from build123d import *

# Parameters (mm, degrees)
SKETCH1_R           = 14.2875
SKETCH1_R_2         = 2.54
BOSS_EXTRUDE1_DEPTH = 3.175
CUT_EXTRUDE1_DEPTH  = 162.674043733
FILLET3_R           = 6.35
SKETCH3_R           = 2.54
BOSS_EXTRUDE3_DEPTH = 3.175
SKETCH6_R           = 2.54
BOSS_EXTRUDE4_DEPTH = 3.175
FILLET2_R           = 6.35
CUT_EXTRUDE2_DEPTH  = 169.237022961
CUT_EXTRUDE3_DEPTH  = 169.237022961
CUT_EXTRUDE4_DEPTH  = 168.265702461
SKETCH15_R          = 2.54
BOSS_EXTRUDE8_DEPTH = 3.175
FILLET4_R           = 2.54


with BuildPart() as part:
    # Sketch1 → Boss-Extrude1 (new body)
    with BuildSketch(Plane.XY):
        with BuildLine():
            Line((-8.89, 25.4), (8.89, 25.4))
            ThreePointArc((8.89, 25.4), (17.870256121, 21.680256121), (21.59, 12.7))
            Line((21.59, 12.7), (21.59, -117.775079775))
            ThreePointArc((21.59, -117.775079775), (21.127743647, -120.388718212), (19.797058824, -122.685251408))
            Line((19.797058824, -122.685251408), (-7.952696208, -155.616779465))
            ThreePointArc((-7.952696208, -155.616779465), (-12.268297602, -157.851943494), (-16.900388255, -156.380852124))
            Line((-16.900388255, -156.380852124), (-32.439211784, -143.287061102))
            ThreePointArc((-32.439211784, -143.287061102), (-34.674375812, -138.971459708), (-33.203284443, -134.339369055))
            Line((-33.203284443, -134.339369055), (-23.382941176, -122.685251408))
            ThreePointArc((-23.382941176, -122.685251408), (-22.052256353, -120.388718212), (-21.59, -117.775079775))
            Line((-21.59, -117.775079775), (-21.59, 12.7))
            ThreePointArc((-21.59, 12.7), (-17.870256121, 21.680256121), (-8.89, 25.4))
        make_face()
        Circle(SKETCH1_R, mode=Mode.SUBTRACT)
        with Locations((0, -101.6)):
            Circle(SKETCH1_R, mode=Mode.SUBTRACT)
        with Locations((-18.532085478, -142.550133084)):
            Circle(SKETCH1_R_2, mode=Mode.SUBTRACT)
        with Locations((0, -50.8)):
            Circle(SKETCH1_R_2, mode=Mode.SUBTRACT)
    extrude(amount=BOSS_EXTRUDE1_DEPTH)

    # Sketch2 → Cut-Extrude1 (cut, through all)
    with BuildSketch(Plane.XY):
        with BuildLine():
            ThreePointArc((19.159083004, -91.647229609), (9.182340769, -50.8), (19.159083004, -9.952770391))
            ThreePointArc((19.159083004, -9.952770391), (20.973467787, -5.122670102), (21.59, 0))
            Line((21.59, 0), (27.94, 0))
            Line((27.94, 0), (27.94, -121.656687185))
            Line((27.94, -121.656687185), (-7.620284479, -163.8572221))
            Line((-7.620284479, -163.8572221), (-17.501317584, -155.874478972))
            Line((-17.501317584, -155.874478972), (16.51, -115.512152961))
            ThreePointArc((16.51, -115.512152961), (20.280273667, -109.005308906), (21.59, -101.6))
            ThreePointArc((21.59, -101.6), (20.973467787, -96.477329898), (19.159083004, -91.647229609))
        make_face()
        with BuildLine():
            Line((-21.59, -41.275), (-21.59, -60.325))
            ThreePointArc((-21.59, -60.325), (-12.065, -50.8), (-21.59, -41.275))
        make_face()
    extrude(amount=CUT_EXTRUDE1_DEPTH, mode=Mode.SUBTRACT)


with BuildPart() as cut_extrude1_piece_1:
    # of the separate pieces the step leaves, piece 1, a body of its own (cut_extrude1_pieces)
    add(part.part.solids().sort_by_distance((-8.89, 25.4, 0))[0])

    # Fillet3
    fillet3_edges = [cut_extrude1_piece_1.edges().sort_by_distance(p)[0] for p in [
        (-21.59, -41.275, 1.5875),
        (-21.59, -60.325, 1.5875),
    ]]
    fillet(fillet3_edges, radius=FILLET3_R)

    # Sketch3 → Boss-Extrude3 (add)
    with BuildSketch(Plane.XY.offset(3.175)):
        with BuildLine():
            Line((-27.351416194, -127.394768527), (-36.025496499, -137.688579))
            ThreePointArc((-36.025496499, -137.688579), (-37.217489152, -141.441859142), (-35.4063854, -144.93869507))
            Line((-35.4063854, -144.93869507), (-24.403104784, -154.210610454))
            ThreePointArc((-24.403104784, -154.210610454), (-19.771014132, -155.681701823), (-15.455412737, -153.446537795))
            Line((-15.455412737, -153.446537795), (-7.557639641, -144.073996091))
            Line((-7.557639641, -144.073996091), (-27.351416194, -127.394768527))
        make_face()
        with Locations((-18.532085478, -142.550133084)):
            Circle(SKETCH3_R, mode=Mode.SUBTRACT)
    extrude(amount=-BOSS_EXTRUDE3_DEPTH)

    # Sketch6 → Boss-Extrude4 (add)
    with BuildSketch(Plane.XY.offset(3.175)):
        Polygon((-35.4063854, -144.93869507), (-63.620410749, -121.164144113), (-51.344981666, -106.596497054), (-27.065569901, -127.055545526), align=None)
        with Locations((-52.626813855, -117.972130278)):
            Circle(SKETCH6_R, mode=Mode.SUBTRACT)
    extrude(amount=-BOSS_EXTRUDE4_DEPTH)

    # Fillet2
    fillet2_edges = [cut_extrude1_piece_1.edges().sort_by_distance(p)[0] for p in [
        (-63.620410749, -121.164144113, 1.5875),
        (-51.344981666, -106.596497054, 1.5875),
        (-27.065569901, -127.055545526, 1.5875),
    ]]
    fillet(fillet2_edges, radius=FILLET2_R)

    # Sketch7 → Cut-Extrude2 (cut, through all)
    with BuildSketch(Plane.XY.offset(3.175)):
        with BuildLine():
            Line((-21.59, 0), (-21.59, 31.75))
            Line((-21.59, 31.75), (21.59, 31.75))
            Line((21.59, 31.75), (21.59, 0))
            ThreePointArc((21.59, 0), (0, 21.59), (-21.59, 0))
        make_face()
    extrude(amount=-CUT_EXTRUDE2_DEPTH, mode=Mode.SUBTRACT)


with BuildPart() as cut_extrude1_piece_2:
    # of the separate pieces the step leaves, piece 2, a body of its own (cut_extrude1_pieces)
    add(part.part.solids().sort_by_distance((-16.900388255, -156.380852124, 0))[0])


with BuildPart() as cut_extrude3_tool:
    # Sketch10 → Cut-Extrude3 (new, through all)
    with BuildSketch(Plane.XY.offset(3.175)):
        with BuildLine():
            Line((-18.151882461, -155.32628042), (-17.361482582, -157.512020269))
            Line((-17.361482582, -157.512020269), (-14.375706423, -156.432313955))
            Line((-14.375706423, -156.432313955), (-15.455412737, -153.446537795))
            ThreePointArc((-15.455412737, -153.446537795), (-16.679911193, -154.563907595), (-18.151882461, -155.32628042))
        make_face()
    extrude(amount=-CUT_EXTRUDE3_DEPTH)


with BuildPart() as cut_extrude1_piece_1_1:
    add(cut_extrude1_piece_1.part)

    # Cut-Extrude3: cut by cut_extrude3_tool
    add(cut_extrude3_tool.part, mode=Mode.SUBTRACT)

    # Sketch12 → Cut-Extrude4 (cut, through all)
    with BuildSketch(Plane.XY.offset(3.175)):
        with BuildLine():
            Line((-21.59, -101.6), (-72.39, -101.6))
            Line((-72.39, -101.6), (-72.39, -165.1))
            Line((-72.39, -165.1), (16.51, -165.1))
            Line((16.51, -165.1), (16.51, -115.512152961))
            ThreePointArc((16.51, -115.512152961), (-7.405308906, -121.880273667), (-21.59, -101.6))
        make_face()
    extrude(amount=-CUT_EXTRUDE4_DEPTH, mode=Mode.SUBTRACT)

    # Sketch15 → Boss-Extrude8 (add)
    with BuildSketch(Plane.XY.offset(3.175)):
        with BuildLine():
            ThreePointArc((-34.29, -3.81), (-30.887045256, -16.51), (-21.59, -25.807045256))
            Line((-21.59, -25.807045256), (-21.59, 0))
            ThreePointArc((-21.59, 0), (-15.266435406, 15.266435406), (0, 21.59))
            Line((0, 21.59), (-8.89, 21.59))
            ThreePointArc((-8.89, 21.59), (-26.850512242, 14.150512242), (-34.29, -3.81))
        make_face()
        with Locations((-24.765, -3.81)):
            Circle(SKETCH15_R, mode=Mode.SUBTRACT)
    extrude(amount=-BOSS_EXTRUDE8_DEPTH)

    # Fillet4
    fillet4_edges = [cut_extrude1_piece_1_1.edges().sort_by_distance(p)[0] for p in [
        (-21.59, -25.807045256, 1.5875),
    ]]
    fillet(fillet4_edges, radius=FILLET4_R)


with BuildPart() as cut_extrude1_piece_2_1:
    add(cut_extrude1_piece_2.part)

    # Cut-Extrude3: cut by cut_extrude3_tool
    add(cut_extrude3_tool.part, mode=Mode.SUBTRACT)


solid = cut_extrude1_piece_1_1.part
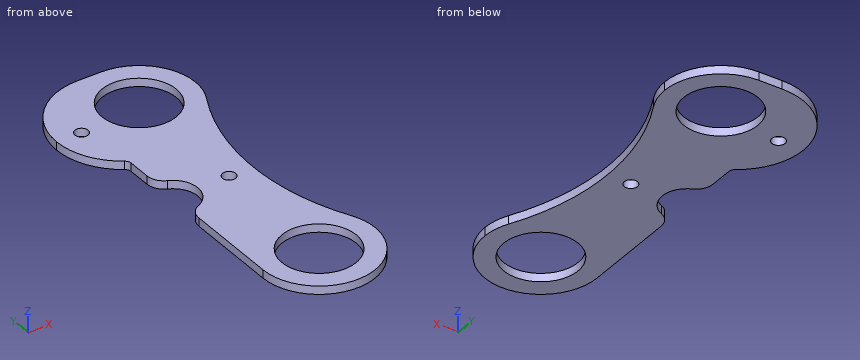
Geometry: final body of the model. Coordinates: model frame, mm. Give positions to 0.01 mm unless a question says otherwise; leave off trailing zeros. Write each loop counter-clockwise with the first axis right and the second up, starting at its lowest first coordinate (ties: lowest second). Pieces come first, ordered by that corner, then holes. Notation, with made-up numbers: M 78,86.25 L 91,86.25 A17 ccw 91,98.25 Z; hole C 1.25,-23.5 d11. An arc over 180 degrees is marked long. Answer in a Markdown table with one row per item. Add a question column.
(1) Section C-C on x = -7.5. Return loops of the section in (y, z) (3 decimals), and give its area (3 significant figures).
(2) Section B-B on z = 2.45. State how many separate pieces and enclosed holes the cut face has, and give its area (3 significant figures).
(3) Ray query, line 1 (Y direction, x = -5.5, z = 0.25); line 2 (Y direction, x = 8, z = 2.4); line 3 (Y direction, x = -19, z = 1.3). Return the intervals inside material, ascending.
(4) Section D-D on x = 5. Return loops of the section in (y, z) (3 decimals).
(5) Section A-A on y = -50.8. Return loops of the section in (x, z) (3 decimals), and give its area (3 significant figures).
(6) First-contact query: pin 1 (1 mm diameter, centred on y = -34.5, z = 1.5, fed in from +X); pin 2 (1.6 mm diameter, centred on y = -82.5, z = 1, fed in from -X); pin 3 (1.5 mm diameter, centred on x = 1.5, z = 2.5, fed in from -Y); pin 4 (4 mm diameter, centred on x = -24.765, y = -3.81, fed in from +Z). Flat tips, straight axial feed; report the tip coordinate or a pass-through.
Result set:
| question | item | result |
|---|---|---|
| 1 | outline | M -121.845,0 L -113.761,0 L -113.761,3.175 L -121.845,3.175 Z; M -89.439,0 L -12.161,0 L -12.161,3.175 L -89.439,3.175 Z; M 12.161,0 L 21.59,0 L 21.59,3.175 L 12.161,3.175 Z |
| 1 | area | 301 mm^2 |
| 2 | separate pieces | 1 |
| 2 | enclosed holes | 4 |
| 2 | area | 4,100 mm^2 |
| 3 | line 1 | y = -122.48 to -114.79, -88.41 to -13.19, 13.19 to 21.59 |
| 3 | line 2 | y = -121.65 to -113.44, -89.76 to -11.84, 11.84 to 20.05 |
| 3 | line 3 | y = -111.85 to -60.23, -41.37 to 19.49 |
| 4 | outline | M -122.603,0 L -114.984,0 L -114.984,3.175 L -122.603,3.175 Z; M -88.216,0 L -13.384,0 L -13.384,3.175 L -88.216,3.175 Z; M 13.384,0 L 21.003,0 L 21.003,3.175 L 13.384,3.175 Z |
| 5 | outline | M -12.065,0 L -2.54,0 L -2.54,3.175 L -12.065,3.175 Z; M 2.54,0 L 9.182,0 L 9.182,3.175 L 2.54,3.175 Z |
| 5 | area | 51.3 mm^2 |
| 6 | pin 1 | stops at x = 10.79 |
| 6 | pin 2 | stops at x = -21.59 |
| 6 | pin 3 | stops at y = -123.18 |
| 6 | pin 4 | passes through |
